For this review, take the finished solid that the model builds, in its own axes (mm). Face numbers are marked on the shaded views. A direction names the side the tool comes from. Coordinates: 2 decimals unless noted, no trailing zeros. Order: outer loops, then holes, each group sorted by start corner. A loop starts at its lowest first (then second) coordinate and runs counter-clockwise, first axis right, second up. Notation, with made-up numbers: (-33.5, 69) -> (25.5, 69) arc R16 ccw to (25.5, 99) -> close; hole circle Ø4 at (-27.5, 85.25). An arc over 180 degrees is marked (long way). Return JSON: item names as keys, results as strings. Group by question number.
Item 1: Draft analysis for pull direction Y (two halves, no side actions). For the marked faces 3, 4 and 5, state which applies: +Y half, -Y half, draft (parallel to the pull), parting line (faces both ways), or undercut.
Item 2: Take a section at D-D (z = 8). Write out the cut boundary in (x, y).
Item 3: Insertion check: pin 1 (5 mm diameter, centred on x = -26, z = 33, fed in from +Y); pin 2 (3.5 mm diameter, centred on x = -26, z = 7, fed in from +Y); pin 3 (1.8 mm diameter, centred on x = 26.5, z = 33, fed in from -Y). Each pin has a flat end and moves straight along its axis. Give the tip position at first contact, or say it passes through.
Item 4: Take a section at C-C (x = 0). Write out the cut boundary in (y, z), then the cut area to 3 significant figures.
Item 5: Take a section at B-B (z = 21). Write out the cut boundary in (x, y).
Item 6: Machinability: for the marked faces 1 and 2, which of the approach directions +Z, -Z, +X, -X, +Y, -Y give a long, thin tool a straight path to every point of the face, cutting with its end or side? Answer none if there is none.
Item 7: Take a section at A-A (y = -12). Write out the cut boundary in (x, z).
Item 8: For line 1 along Z through (x, y) = (-26, -17); line 2 along Y through (x, z) = (17, 23); line 3 along Y through (x, z) = (-17.5, 28), list the stretches that pass through material, from the lowest coordinate up.
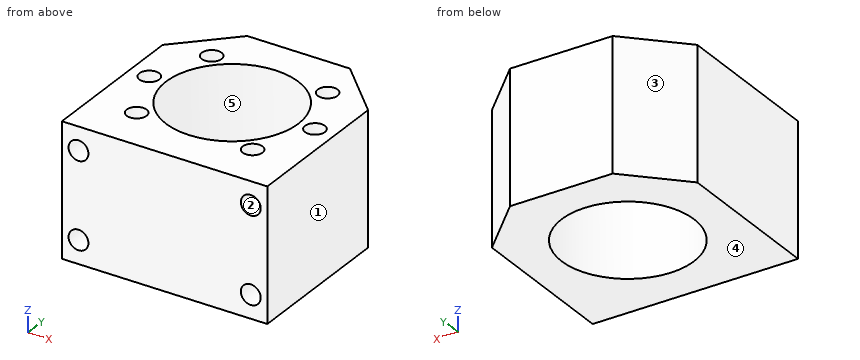
```python
from build123d import *

# Parameters (mm, degrees)
DODANIE_WYCI_GNI_CIE1_DEPTH = 40
SZKIC2_R                    = 20
WYTNIJ_WYCI_GNI_CIE1_DEPTH  = 40
SZKIC4_R                    = 3
WYTNIJ_WYCI_GNI_CIE2_DEPTH  = 25
SZKIC5_R                    = 3
WYTNIJ_WYCI_GNI_CIE4_DEPTH  = 25


with BuildPart() as part:
    # Szkic1 → Dodanie-wyciągnięcie1 (new body)
    with BuildSketch(Plane.XY):
        Polygon((31, -31.5), (31, 15.5), (15.5, 31), (-15.5, 31), (-31, 15.5), (-31, -31.5), align=None)
    extrude(amount=DODANIE_WYCI_GNI_CIE1_DEPTH)

    # Szkic2 → Wytnij-wyciągnięcie1 (cut)
    with BuildSketch(Plane.XY.offset(40)):
        Circle(SZKIC2_R)
    extrude(amount=-WYTNIJ_WYCI_GNI_CIE1_DEPTH, mode=Mode.SUBTRACT)

    # Szkic4 → Wytnij-wyciągnięcie2 (cut)
    with BuildSketch(Plane.XY.offset(40)):
        with Locations((17.5, -17.5)):
            Circle(SZKIC4_R)
        with Locations((25, 0)):
            Circle(SZKIC4_R)
        with Locations((17.5, 17.5)):
            Circle(SZKIC4_R)
        with Locations((-25, 0)):
            Circle(SZKIC4_R)
        with Locations((-17.5, 17.5)):
            Circle(SZKIC4_R)
        with Locations((-17.5, -17.5)):
            Circle(SZKIC4_R)
    extrude(amount=-WYTNIJ_WYCI_GNI_CIE2_DEPTH, mode=Mode.SUBTRACT)

    # Szkic5 → Wytnij-wyciągnięcie4 (cut)
    with BuildSketch(Plane.XZ.offset(31.5)):
        with Locations((-26, 33)):
            Circle(SZKIC5_R)
        with Locations((-26, 7)):
            Circle(SZKIC5_R)
        with Locations((26, 33)):
            Circle(SZKIC5_R)
        with Locations((26, 7)):
            Circle(SZKIC5_R)
    extrude(amount=-WYTNIJ_WYCI_GNI_CIE4_DEPTH, mode=Mode.SUBTRACT)


solid = part.part
```
Findings below:
{
 "1": {"face 3": "+Y half", "face 4": "draft", "face 5": "undercut"},
 "2": {"outline": "(-31, -31.5) -> (-28.83, -31.5) -> (-28.83, -6.5) -> (-23.17, -6.5) -> (-23.17, -31.5) -> (23.17, -31.5) -> (23.17, -6.5) -> (28.83, -6.5) -> (28.83, -31.5) -> (31, -31.5) -> (31, 15.5) -> (15.5, 31) -> (-15.5, 31) -> (-31, 15.5) -> close; hole circle Ø40 at (0, 0)"},
 "3": {"pin 1": "stops at y = 23", "pin 2": "stops at y = 22.25", "pin 3": "stops at y = -6.5"},
 "4": {"outline": "(-31.5, 0) -> (-20, 0) -> (-20, 40) -> (-31.5, 40) -> close; (20, 0) -> (31, 0) -> (31, 40) -> (20, 40) -> close", "area": "900 mm2"},
 "5": {"outline": "(-31, -31.5) -> (31, -31.5) -> (31, 15.5) -> (15.5, 31) -> (-15.5, 31) -> (-31, 15.5) -> close; hole circle Ø6 at (-25, 0); hole circle Ø6 at (-17.5, -17.5); hole circle Ø6 at (-17.5, 17.5); hole circle Ø40 at (0, 0); hole circle Ø6 at (17.5, -17.5); hole circle Ø6 at (17.5, 17.5); hole circle Ø6 at (25, 0)"},
 "6": {"face 1": "+Z, -Z, +X, +Y, -Y", "face 2": "-Y"},
 "7": {"outline": "(-31, 0) -> (-16, 0) -> (-16, 40) -> (-31, 40) -> close; (16, 0) -> (31, 0) -> (31, 40) -> (16, 40) -> close; hole circle Ø6 at (-26, 7); hole circle Ø6 at (-26, 33); hole circle Ø6 at (26, 7); hole circle Ø6 at (26, 33)"},
 "8": {"line 1": "z = 0 to 4, 10 to 30, 36 to 40", "line 2": "y = -31.5 to -20.46, -14.54 to -10.54, 10.54 to 14.54, 20.46 to 29.5", "line 3": "y = -31.5 to -20.5, -14.5 to -9.68, 9.68 to 14.5, 20.5 to 29"}
}
